from build123d import *

# Parameters (mm, degrees)
SKETCH_1_R          = 21
SKETCH_1_R_2        = 13.5
EXTRUDE_1_DEPTH     = 5
SKETCH_4_R          = 1.45
CUT_EXTRUDE_1_DEPTH = 420.336678577
SKETCH_5_R          = 1.95
CUT_EXTRUDE_2_DEPTH = 420.336678577
CUT_EXTRUDE_3_DEPTH = 420.336678577


with BuildPart() as part:
    # 草图1 → 凸台-拉伸1 (new body)
    with BuildSketch(Plane.XY):
        with BuildLine():
            Line((400.346875, 18.496747761), (0.4875, 25.995429286))
            ThreePointArc((0.4875, 25.995429286), (-26, 0), (0.4875, -25.995429286))
            Line((0.4875, -25.995429286), (400.346875, -18.496747761))
            ThreePointArc((400.346875, -18.496747761), (418.5, 0), (400.346875, 18.496747761))
        make_face()
        Circle(SKETCH_1_R, mode=Mode.SUBTRACT)
        with Locations((400, 0)):
            Circle(SKETCH_1_R_2, mode=Mode.SUBTRACT)
    extrude(amount=EXTRUDE_1_DEPTH)

    # 草图4 → 切除-拉伸1 (cut, through all)
    with BuildSketch(Plane(origin=(0, 0, 0), x_dir=(-1, 0, 0), z_dir=(0, 0, -1))):
        with Locations((-40.693979899, -5)):
            Circle(SKETCH_4_R)
        with Locations(Location((-40.693979899, 5, 0), (0, 0, 180))):
            Circle(SKETCH_4_R)
    extrude(amount=-CUT_EXTRUDE_1_DEPTH, mode=Mode.SUBTRACT)

    # 草图5 → 切除-拉伸2 (cut, through all)
    with BuildSketch(Plane(origin=(0, 0, 0), x_dir=(-1, 0, 0), z_dir=(0, 0, -1))):
        with Locations((-200, 5)):
            Circle(SKETCH_5_R)
        with Locations(Location((-200, -5, 0), (0, 0, 180))):
            Circle(SKETCH_5_R)
    extrude(amount=-CUT_EXTRUDE_2_DEPTH, mode=Mode.SUBTRACT)

    # 草图6 → 切除-拉伸3 (cut, through all)
    with BuildSketch(Plane.XY.offset(5)):
        with BuildLine():
            Line((50.750229899, 17.051430775), (190.05625, 14.438983638))
            ThreePointArc((190.05625, 14.438983638), (192.99947261, 11.383261028), (189.94375, 8.440038418))
            Line((189.94375, 8.440038418), (50.637729899, 11.052485555))
            ThreePointArc((50.637729899, 11.052485555), (47.694507289, 14.108208165), (50.750229899, 17.051430775))
        make_face()
        with BuildLine():
            Line((210.075, 15.063741906), (375.075, 11.969447939))
            ThreePointArc((375.075, 11.969447939), (378.999296813, 7.895151126), (374.925, 3.970854313))
            Line((374.925, 3.970854313), (209.925, 7.06514828))
            ThreePointArc((209.925, 7.06514828), (206.000703187, 11.139445093), (210.075, 15.063741906))
        make_face()
        with BuildLine():
            Line((210.075, -15.063741906), (375.075, -11.969447939))
            ThreePointArc((375.075, -11.969447939), (378.999296813, -7.895151126), (374.925, -3.970854313))
            Line((374.925, -3.970854313), (209.925, -7.06514828))
            ThreePointArc((209.925, -7.06514828), (206.000703187, -11.139445093), (210.075, -15.063741906))
        make_face()
        with BuildLine():
            Line((50.750229899, -17.051430775), (190.05625, -14.438983638))
            ThreePointArc((190.05625, -14.438983638), (192.99947261, -11.383261028), (189.94375, -8.440038418))
            Line((189.94375, -8.440038418), (50.637729899, -11.052485555))
            ThreePointArc((50.637729899, -11.052485555), (47.694507289, -14.108208165), (50.750229899, -17.051430775))
        make_face()
        with BuildLine():
            Line((50.693979899, 4), (190, 4))
            ThreePointArc((190, 4), (194, 0), (190, -4))
            Line((190, -4), (50.693979899, -4))
            ThreePointArc((50.693979899, -4), (46.693979899, 0), (50.693979899, 4))
        make_face()
    extrude(amount=-CUT_EXTRUDE_3_DEPTH, mode=Mode.SUBTRACT)


solid = part.part
Work out the finished part from the listing and answer in its coordinate system (mm). Give positions to 0.01 mm unless a question says otherwise; leave off trailing zeros. Write each loop counter-clockwise with the first axis right and the second up, starting at its lowest first coordinate (ties: lowest second). Pieces come first, ordered by that corner, then holes. Notation, with made-up numbers: M 70.5,59.5 L 116.5,59.5 A31 ccw 116.5,85.5 Z; hole C -24,84.5 d3. An arc over 180 degrees is marked long. Answer as CSV lines item,"result".
Q1. A cutting plane is placed at C-C on x = 120. Write down the section's boundary in (y, z).
A:
outline,"M -23.75,0 L -15.75,0 L -15.75,5 L -23.75,5 Z; M -9.75,0 L -4,0 L -4,5 L -9.75,5 Z; M 4,0 L 9.75,0 L 9.75,5 L 4,5 Z; M 15.75,0 L 23.75,0 L 23.75,5 L 15.75,5 Z"
Q2. A cutting plane is placed at A-A on z = 3.65. Count the separate pieces of the cut face and the enclosed holes in it, plus the area to 3 significant figures.
A:
separate pieces,"1"
enclosed holes,"11"
area,"11,800 mm²"
Q3. Given P1, Ø25, axis at x = 0, y = 0, coming from the -Z side; P2, Ø2, axis at x = 21, z = 1.5, coming from the -Y side, each flat-ended and moving along its own axis, determine where each tip first touches the part or whether it passes through.
A:
P1,"passes through"
P2,"stops at y = -25.63"
Q4. A cutting plane is placed at B-B on x = 288.5. Write down the section's boundary in (y, z), plus the area to 3 significant figures.
A:
outline,"M -20.59,0 L -13.59,0 L -13.59,5 L -20.59,5 Z; M -5.59,0 L 5.59,0 L 5.59,5 L -5.59,5 Z; M 13.59,0 L 20.59,0 L 20.59,5 L 13.59,5 Z"
area,"126 mm²"
Q5. A cutting plane is placed at D-D on x = 10.5. Write down the section's boundary in (y, z), plus the area to 3 significant figures.
A:
outline,"M -25.81,0 L -18.19,0 L -18.19,5 L -25.81,5 Z; M 18.19,0 L 25.81,0 L 25.81,5 L 18.19,5 Z"
area,"76.2 mm²"
Q6. Find the intervals of material crossed by probe 1 along Y at (x, z) = (329.5, 2.4); probe 2 along X at (y, z) = (7.5, 1.65); probe 3 along Y at (x, z) = (155.5, 2.25), in increasing order. Write a range as [from, to].
A:
probe 1,"y = [-19.83, -12.82], [-4.82, 4.82], [12.82, 19.83]"
probe 2,"x = [-24.89, -19.62], [19.62, 208.18], [378.97, 388.78], [411.22, 416.91]"
probe 3,"y = [-23.09, -15.09], [-9.09, -4], [4, 9.09], [15.09, 23.09]"
Q7. The mould has two halves that part along Y. Classify faces 1 (the flat face through (193, -5, 0)), 2 (the cylindrical face through (-25.994, 0.579, 2.465)), 3 (the cylindrical face through (412.47, -5.17, 2.46)): +Y half, -Y half, draft (parallel to the pull), parting line (faces both ways), or undercut.
A:
face 1,"draft"
face 2,"parting line"
face 3,"undercut"
